Build history of the part. All positions in model axes, mm. Face numbers are marked on the shaded views. A direction names the side the tool comes from. Round coordinates to 2 decimals unless told otherwise and drop trailing zeros. Write each loop counter-clockwise with the first axis right and the second up, starting at its lowest first coordinate (ties: lowest second). Pieces come first, ordered by that corner, then holes.
1) Saw through at C-C (z = -10). Write the cut outline in (x, y).
2) Saw through at D-D (y = 2). Write the cut outline in (x, z) (3 decimals).
3) Wall check: probe 1 along Z at (x, y) = (30.48, 10.5) (3 decimals); probe 2 along X at (y, z) = (-44, -24.5); probe 3 along X at (y, z) = (1.5, -23). Give the ranges that are in metal, low to high.
4) Pull direction Z, two halves, no side cores. Call the marked faces 1, 2 and 3: +Z half, -Z half, draft (parallel to the pull), parting line (faces both ways), or undercut.
5) Saw through at B-B (x = 0). Write the cut outline in (y, z), plus the area to 3 significant figures.
6) Flat gauge pins, fed straight in: pin 1 (4 mm diameter, centred on y = 11.5, z = -2.5, fed in from -X); pin 2 (3 mm diameter, centred on x = -9.5, z = -17.5, fed in from -Y); pin 3 (1.9 mm diameter, centred on y = 12.5, z = 27.5, fed in from +X). Where does each tip first touch, or does it go through?
7) Saw through at A-A (y = -36). Write the cut outline in (x, z), plus the area to 3 significant figures.
8) Which spindle directions (+Z, -Z, +X, -X, +Y, -Y) get a long thin tool onto all of the face, cutting with end or side? Do the marked faces 4, 5 and 6. Say none if no direction does.
from build123d import *

# Parameters (mm, degrees)
BOSS_EXTRUDE1_DEPTH = 31.75
CUT_EXTRUDE1_DEPTH  = 118.537522281
CUT_EXTRUDE2_DEPTH  = 7.62
SKETCH5_W           = 24.13
SKETCH5_H           = 3.81
CUT_EXTRUDE3_DEPTH  = 95.766937067
CUT_EXTRUDE4_REACH  = 84.159
SKETCH6_R           = 12.7
CUT_EXTRUDE5_REACH  = 89.52
SKETCH7_R           = 3.81


with BuildPart() as part:
    # Sketch2 → Boss-Extrude1 (new, symmetric)
    with BuildSketch(Plane.XY):
        with BuildLine():
            Line((-29.591, 0), (29.591, 0))
            ThreePointArc((29.591, 0), (37.673230509, -3.347769491), (41.021, -11.43))
            Line((41.021, -11.43), (41.021, -48.26))
            Line((41.021, -48.26), (51.181, -48.26))
            Line((51.181, -48.26), (51.181, -11.43))
            ThreePointArc((51.181, -11.43), (49.29585059, -1.827302371), (43.920228208, 6.35))
            ThreePointArc((43.920228208, 6.35), (41.232417018, 10.438651186), (40.289842313, 15.24))
            Line((40.289842313, 15.24), (-40.289842313, 15.24))
            ThreePointArc((-40.289842313, 15.24), (-41.232417018, 10.438651186), (-43.920228208, 6.35))
            ThreePointArc((-43.920228208, 6.35), (-49.29585059, -1.827302371), (-51.181, -11.43))
            Line((-51.181, -11.43), (-51.181, -48.26))
            Line((-51.181, -48.26), (-41.021, -48.26))
            Line((-41.021, -48.26), (-41.021, -11.43))
            ThreePointArc((-41.021, -11.43), (-37.673230509, -3.347769491), (-29.591, 0))
        make_face()
    extrude(amount=BOSS_EXTRUDE1_DEPTH, both=True)

    # Sketch3 → Cut-Extrude1 (cut, through all)
    with BuildSketch(Plane(origin=(51.181, 0, 0), x_dir=(0, 0, -1), z_dir=(1, 0, 0))):
        with BuildLine():
            Line((-17.78, -48.26), (17.78, -48.26))
            Line((17.78, -48.26), (17.78, -29.21))
            ThreePointArc((17.78, -29.21), (0, -11.43), (-17.78, -29.21))
            Line((-17.78, -29.21), (-17.78, -48.26))
        make_face()
    extrude(amount=-CUT_EXTRUDE1_DEPTH, mode=Mode.SUBTRACT)

    # Sketch4 → Cut-Extrude2 (cut)
    with BuildSketch(Plane(origin=(0, 15.24, 0), x_dir=(1, 0, 0), z_dir=(0, 1, 0))):
        with BuildLine():
            Line((-20.223842313, 19.304), (20.223842313, 19.304))
            ThreePointArc((20.223842313, 19.304), (22.738314027, 18.262471714), (23.779842313, 15.748))
            Line((23.779842313, 15.748), (23.779842313, -15.748))
            ThreePointArc((23.779842313, -15.748), (22.738314027, -18.262471714), (20.223842313, -19.304))
            Line((20.223842313, -19.304), (-20.223842313, -19.304))
            ThreePointArc((-20.223842313, -19.304), (-22.738314027, -18.262471714), (-23.779842313, -15.748))
            Line((-23.779842313, -15.748), (-23.779842313, 15.748))
            ThreePointArc((-23.779842313, 15.748), (-22.738314027, 18.262471714), (-20.223842313, 19.304))
        make_face()
    extrude(amount=-CUT_EXTRUDE2_DEPTH, mode=Mode.SUBTRACT)

    # Sketch5 → Cut-Extrude3 (cut, through all)
    with BuildSketch(Plane.XY.offset(31.75)):
        with Locations((0, 13.335)):
            Rectangle(SKETCH5_W, SKETCH5_H)
    extrude(amount=-CUT_EXTRUDE3_DEPTH, mode=Mode.SUBTRACT)

    # Sketch6 → Cut-Extrude4 (cut, up to next)
    with BuildSketch(Plane(origin=(0, 7.62, 0), x_dir=(1, 0, 0), z_dir=(0, 1, 0)), mode=Mode.PRIVATE) as cut_extrude4_sk1:
        with Locations(Location((0, 0, 0), (0, 0, 270))):
            Circle(SKETCH6_R)
    cut_extrude4_tool1 = extrude(cut_extrude4_sk1.sketch, amount=-CUT_EXTRUDE4_REACH, mode=Mode.PRIVATE) & part.part
    add(cut_extrude4_tool1.solids().sort_by_distance((0, 7.62, 0))[0], mode=Mode.SUBTRACT)

    # Sketch7 → Cut-Extrude5 (cut, up to next)
    with BuildSketch(Plane(origin=(0, 15.24, 0), x_dir=(1, 0, 0), z_dir=(0, 1, 0)), mode=Mode.PRIVATE) as cut_extrude5_sk1:
        with Locations(Location((-30.48, 22.225, 0), (0, 0, 270))):
            Circle(SKETCH7_R)
    cut_extrude5_tool1 = extrude(cut_extrude5_sk1.sketch, amount=-CUT_EXTRUDE5_REACH, mode=Mode.PRIVATE) & part.part
    # Sketch7 → Cut-Extrude5 (cut, up to next)
    with BuildSketch(Plane(origin=(0, 15.24, 0), x_dir=(1, 0, 0), z_dir=(0, 1, 0)), mode=Mode.PRIVATE) as cut_extrude5_sk2:
        with Locations(Location((30.48, 22.225, 0), (0, 0, 270))):
            Circle(SKETCH7_R)
    cut_extrude5_tool2 = extrude(cut_extrude5_sk2.sketch, amount=-CUT_EXTRUDE5_REACH, mode=Mode.PRIVATE) & part.part
    # Sketch7 → Cut-Extrude5 (cut, up to next)
    with BuildSketch(Plane(origin=(0, 15.24, 0), x_dir=(1, 0, 0), z_dir=(0, 1, 0)), mode=Mode.PRIVATE) as cut_extrude5_sk3:
        with Locations(Location((30.48, -22.225, 0), (0, 0, 270))):
            Circle(SKETCH7_R)
    cut_extrude5_tool3 = extrude(cut_extrude5_sk3.sketch, amount=-CUT_EXTRUDE5_REACH, mode=Mode.PRIVATE) & part.part
    # Sketch7 → Cut-Extrude5 (cut, up to next)
    with BuildSketch(Plane(origin=(0, 15.24, 0), x_dir=(1, 0, 0), z_dir=(0, 1, 0)), mode=Mode.PRIVATE) as cut_extrude5_sk4:
        with Locations(Location((-30.48, -22.225, 0), (0, 0, 270))):
            Circle(SKETCH7_R)
    cut_extrude5_tool4 = extrude(cut_extrude5_sk4.sketch, amount=-CUT_EXTRUDE5_REACH, mode=Mode.PRIVATE) & part.part
    add(cut_extrude5_tool1.solids().sort_by_distance((-30.48, 15.24, -22.225))[0], mode=Mode.SUBTRACT)
    add(cut_extrude5_tool2.solids().sort_by_distance((30.48, 15.24, -22.225))[0], mode=Mode.SUBTRACT)
    add(cut_extrude5_tool3.solids().sort_by_distance((30.48, 15.24, 22.225))[0], mode=Mode.SUBTRACT)
    add(cut_extrude5_tool4.solids().sort_by_distance((-30.48, 15.24, 22.225))[0], mode=Mode.SUBTRACT)


solid = part.part
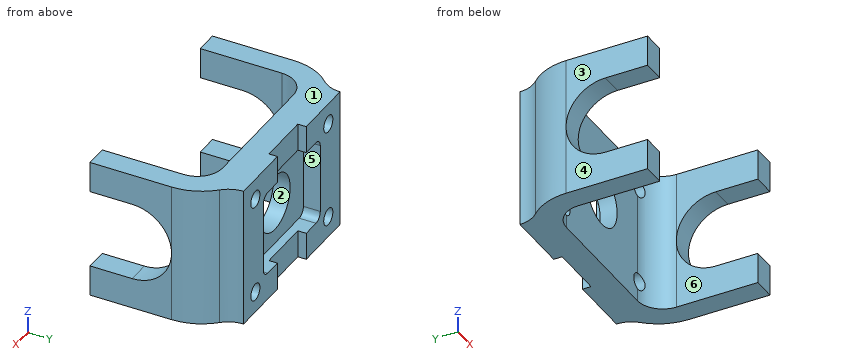
Evaluation:
1. outline: (-51.18, -14.51) - (-41.02, -14.51) - (-41.02, -11.43) arc R11.43 cw to (-29.59, 0) - (-7.83, 0) - (-7.83, 7.62) - (-23.78, 7.62) - (-23.78, 15.24) - (-40.29, 15.24) arc R12.7 cw to (-43.92, 6.35) arc R25.4 ccw to (-51.18, -11.43) - close; (7.83, 0) - (29.59, 0) arc R11.43 cw to (41.02, -11.43) - (41.02, -14.51) - (51.18, -14.51) - (51.18, -11.43) arc R25.4 ccw to (43.92, 6.35) arc R12.7 cw to (40.29, 15.24) - (23.78, 15.24) - (23.78, 7.62) - (7.83, 7.62) - close
2. outline: (-47.34, -31.75) - (47.34, -31.75) - (47.34, 31.75) - (-47.34, 31.75) - close; hole circle Ø7.62 at (-30.48, -22.225); hole circle Ø7.62 at (-30.48, 22.225); hole circle Ø25.4 at (0, 0); hole circle Ø7.62 at (30.48, -22.225); hole circle Ø7.62 at (30.48, 22.225)
3. probe 1: z = -31.75 to -26.035, -18.415 to 18.415, 26.035 to 31.75
3. probe 2: x = -51.18 to -41.02, 41.02 to 51.18
3. probe 3: x = -47.64 to -34.21, -26.75 to 26.75, 34.21 to 47.64
4. face 1: +Z half
4. face 2: undercut
4. face 3: draft
5. outline: (0, -31.75) - (11.43, -31.75) - (11.43, -19.3) - (7.62, -19.3) - (7.62, -12.7) - (0, -12.7) - close; (0, 12.7) - (7.62, 12.7) - (7.62, 19.3) - (11.43, 19.3) - (11.43, 31.75) - (0, 31.75) - close
5. area: 385 mm2
6. pin 1: stops at x = -41.66
6. pin 2: stops at y = 0
6. pin 3: stops at x = 40.84
7. outline: (-51.18, -31.75) - (-41.02, -31.75) - (-41.02, -17.78) - (-51.18, -17.78) - close; (-51.18, 17.78) - (-41.02, 17.78) - (-41.02, 31.75) - (-51.18, 31.75) - close; (41.02, -31.75) - (51.18, -31.75) - (51.18, -17.78) - (41.02, -17.78) - close; (41.02, 17.78) - (51.18, 17.78) - (51.18, 31.75) - (41.02, 31.75) - close
7. area: 568 mm2
8. face 4: +Z, -Z, -X, +Y, -Y
8. face 5: +Y
8. face 6: +Z, -Z, -Y
